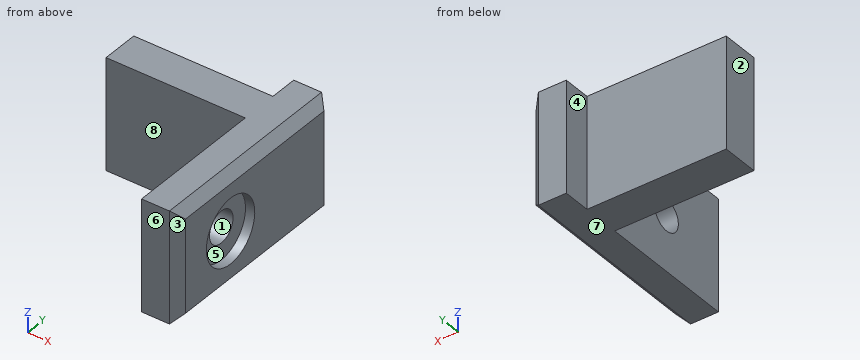
```python
from build123d import *

# Parameters (mm, degrees)
BOSS_EXTRUDE1_DEPTH = 12
SKETCH2_R           = 1.7
CUT_EXTRUDE1_DEPTH  = 12
SKETCH3_R           = 3.5
CUT_EXTRUDE2_DEPTH  = 1
CHAMFER1_SIZE       = 1


with BuildPart() as part:
    # Sketch1 → Boss-Extrude1 (new body)
    with BuildSketch(Plane.XY):
        Polygon((0, 19), (15, 19), (15, 22), (19, 22), (19, 19), (19, 0), (15, 0), (15, 15), (0, 15), align=None)
    extrude(amount=BOSS_EXTRUDE1_DEPTH)

    # Sketch2 → Cut-Extrude1 (cut)
    with BuildSketch(Plane.ZY.offset(-15)):
        with Locations((6, 7.5)):
            Circle(SKETCH2_R)
    extrude(amount=-CUT_EXTRUDE1_DEPTH, mode=Mode.SUBTRACT)

    # Sketch3 → Cut-Extrude2 (cut)
    with BuildSketch(Plane(origin=(19, 0, 0), x_dir=(0, 0, -1), z_dir=(1, 0, 0))):
        with Locations((-6, 7.5)):
            Circle(SKETCH3_R)
    extrude(amount=-CUT_EXTRUDE2_DEPTH, mode=Mode.SUBTRACT)

    # Chamfer1
    chamfer1_edges = [part.edges().sort_by_distance(p)[0] for p in [
        (19, 11, 12),
        (19, 11, 0),
        (19, 22, 6),
        (19, 0, 6),
    ]]
    chamfer(chamfer1_edges, length=CHAMFER1_SIZE)


solid = part.part
```
For this review, take the finished solid that the model builds, in its own axes (mm). Face numbers are marked on the shaded views. A direction names the side the tool comes from. Coordinates: 2 decimals unless noted, no trailing zeros. Write each loop counter-clockwise with the first axis right and the second up, starting at its lowest first coordinate (ties: lowest second). Pieces come first, ordered by that corner, then holes. Notation, with made-up numbers: (37, -12) - (71, -12) arc R8 cw to (71, 1) - close; hole circle Ø3 at (21.25, 19.5). An arc over 180 degrees is marked (long way). Answer in a Markdown table with one row per item. Add a question column.
Q1. We need section A-A, the plane z = 6. State the section outline as (x, y) points.
Q2. For probe 1 along Y at (x, z) = (16.2, 6); probe 2 along Y at (x, z) = (3, 11.25); probe 3 along X at (y, z) = (6.5, 8.25), list the stretches that pass through material, from the lowest coordinate up.
Q3. We need section D-D, the plane y = 13.75. State the section outline as (x, z) points.
Q4. For P1, Ø2, axis at x = 12.5, z = 10, coming from the +Y side; P2, Ø3.5, axis at x = 9.5, z = 6, coming from the -Y side; P3, Ø5.5, axis at y = 7.5, z = 6, coming from the +X side, all flat-tipped, find the tip position at first contact; note any pin that passes through.
Q5. We need section C-C, the plane x = 15.5. State the section outline as (y, z) points.
Q6. Tool access review of the marked faces 4, 5, 6, 7 and 8: name each direction out of +Z, -Z, +X, -X, +Y, -Y from which nothing blocks a thin tool from reaching the whole face with its end or side.
Q7. Draft analysis for pull direction Y (two halves, no side actions). For the marked faces 1, 2 and 3, state which applies: +Y half, -Y half, draft (parallel to the pull), parting line (faces both ways), or undercut.
Q8. We need section B-B, the plane y = 7.5. State the section outline as (x, z) points, and give its area (3 significant figures).
Answer list:
| question | item | result |
|---|---|---|
| 1 | outline | (0, 15) - (15, 15) - (15, 9.2) - (18, 9.2) - (18, 11) - (19, 11) - (19, 21) - (18, 22) - (15, 22) - (15, 19) - (0, 19) - close; (15, 0) - (18, 0) - (19, 1) - (19, 4) - (18, 4) - (18, 5.8) - (15, 5.8) - close |
| 2 | probe 1 | y = 0 to 5.8, 9.2 to 22 |
| 2 | probe 2 | y = 15 to 19 |
| 2 | probe 3 | x = 15 to 18 |
| 3 | outline | (15, 0) - (18, 0) - (19, 1) - (19, 11) - (18, 12) - (15, 12) - close |
| 4 | P1 | stops at y = 19 |
| 4 | P2 | stops at y = 15 |
| 4 | P3 | stops at x = 18 |
| 5 | outline | (0, 0) - (22, 0) - (22, 12) - (0, 12) - close; hole circle Ø3.4 at (7.5, 6) |
| 6 | face 4 | +Z, -Z, -X, +Y |
| 6 | face 5 | +X |
| 6 | face 6 | +Z, -Z, +X, -X, -Y |
| 6 | face 7 | -Z, +X, -X, +Y, -Y |
| 6 | face 8 | +Z, -Z, -X, -Y |
| 7 | face 1 | undercut |
| 7 | face 2 | draft |
| 7 | face 3 | -Y half |
| 8 | outline | (15, 0) - (18, 0) - (19, 1) - (19, 2.5) - (18, 2.5) - (18, 4.3) - (15, 4.3) - close; (15, 7.7) - (18, 7.7) - (18, 9.5) - (19, 9.5) - (19, 11) - (18, 12) - (15, 12) - close |
| 8 | area | 29.8 mm2 |
